```python
from build123d import *

# Parameters (mm, degrees)
SKETCH1_W           = 25
SKETCH1_H           = 200
BOSS_EXTRUDE1_DEPTH = 6
SKETCH2_R           = 2.5
SKETCH2_R_2         = 3
CUT_EXTRUDE1_DEPTH  = 6


with BuildPart() as part:
    # Sketch1 → Boss-Extrude1 (new body)
    with BuildSketch(Plane.XY):
        Rectangle(SKETCH1_W, SKETCH1_H)
    extrude(amount=BOSS_EXTRUDE1_DEPTH)

    # Sketch2 → Cut-Extrude1 (cut)
    with BuildSketch(Plane.XY.offset(6)):
        with Locations((0, -60)):
            Circle(SKETCH2_R)
        with Locations(Location((0, 60, 0), (0, 0, 180))):
            Circle(SKETCH2_R)
        with Locations((0, -40)):
            Circle(SKETCH2_R_2)
        with Locations(Location((0, 40, 0), (0, 0, 180))):
            Circle(SKETCH2_R_2)
    extrude(amount=-CUT_EXTRUDE1_DEPTH, mode=Mode.SUBTRACT)


solid = part.part
```
CAD build for the part. Positions are in the model's coordinates, mm. Round coordinates to 2 decimals unless told otherwise and drop trailing zeros. Loops run counter-clockwise (first coordinate to the right, second up) from the corner with the lowest first, then second, coordinate; pieces in that order, holes last. Notation, with made-up numbers: M 77.5,19.25 L 98.5,19.25 A20 cw 98.5,44.25 Z; hole C 72,32 d9. An arc over 180 degrees is marked long. Use a Markdown table: item, result. Add a question column.
(1) Pull direction X, two halves, no side cores. Call faces 1 (the face through (0, 37, 3)), 2 (the face through (12.5, -1, 3)), 3 (the face through (0, 1, 6)): +X half, -X half, draft (parallel to the pull), parting line (faces both ways), or undercut.
(2) Cut at B-B (x = 0). Give the cut face in (y, z), and give its area (3 significant figures).
(3) Cut at C-C (z = 3.15). Give the cut face in (x, y), and give its area (3 significant figures).
(4) Drill centre lines: line 1 (Y direction, x = 0, z = 1.75); line 2 (Y direction, x = 1, z = 0.5); line 3 (X direction, y = 60, z = 4). Where is each one in solid material? Low to high.
(5) Cut at A-A (y = -60). Give the cut face in (x, z), and give its area (3 significant figures).
Geometry says:
| question | item | result |
|---|---|---|
| 1 | face 1 | undercut |
| 1 | face 2 | +X half |
| 1 | face 3 | draft |
| 2 | outline | M -100,0 L -62.5,0 L -62.5,6 L -100,6 Z; M -57.5,0 L -43,0 L -43,6 L -57.5,6 Z; M -37,0 L 37,0 L 37,6 L -37,6 Z; M 43,0 L 57.5,0 L 57.5,6 L 43,6 Z; M 62.5,0 L 100,0 L 100,6 L 62.5,6 Z |
| 2 | area | 1,070 mm² |
| 3 | outline | M -12.5,-100 L 12.5,-100 L 12.5,100 L -12.5,100 Z; hole C 0,-40 d6; hole C 0,40 d6; hole C 0,-60 d5; hole C 0,60 d5 |
| 3 | area | 4,900 mm² |
| 4 | line 1 | y = -100 to -62.5, -57.5 to -43, -37 to 37, 43 to 57.5, 62.5 to 100 |
| 4 | line 2 | y = -100 to -62.29, -57.71 to -42.83, -37.17 to 37.17, 42.83 to 57.71, 62.29 to 100 |
| 4 | line 3 | x = -12.5 to -2.5, 2.5 to 12.5 |
| 5 | outline | M -12.5,0 L -2.5,0 L -2.5,6 L -12.5,6 Z; M 2.5,0 L 12.5,0 L 12.5,6 L 2.5,6 Z |
| 5 | area | 120 mm² |
